Here's the drawing with two shaded views (mm, measured from the low corner). I have some questions. Give positions to 0.01 mm unless a question says otherwise; leave off trailing zeros. Order: outer loops, then holes, each group sorted by start corner. A loop starts at its lowest first (then second) coordinate and runs counter-clockwise, first axis right, second up. Notation, with made-up numbers: (55, -6.5) - (102, -6.5) arc R16 cw to (102, -1.5) - close; hole circle Ø3 at (-35, 19.5). An arc over 180 degrees is marked (long way). Use one line per item in the form item = value. Start each with the question number.
1) For pin 1 (10 mm diameter, centred on y = 25, z = 12.5, fed in from -X); pin 2 (8 mm diameter, centred on y = 42.5, z = 20.5, fed in from +X) (1 decimal); pin 3 (10 mm diameter, centred on x = 45, z = 3, fed in from +Y); pin 4 (8 mm diameter, centred on y = 9.5, z = 17, fed in from -X), each with a flat end and sliding along its axis, tell me the tip position at first contact or that it passes through.
2) Suppose I cut it at A-A, the plane z = 14. Write out the boundary of the cut face in (x, y) (1 decimal), and give its area (3 significant figures).
3) Please list where these lines run through material, in increasing order: probe 1 along X at (y, z) = (29.5, 8.75) (1 decimal); probe 2 along X at (y, z) = (28.5, 14.25); probe 3 along Y at (x, z) = (37.5, 18).
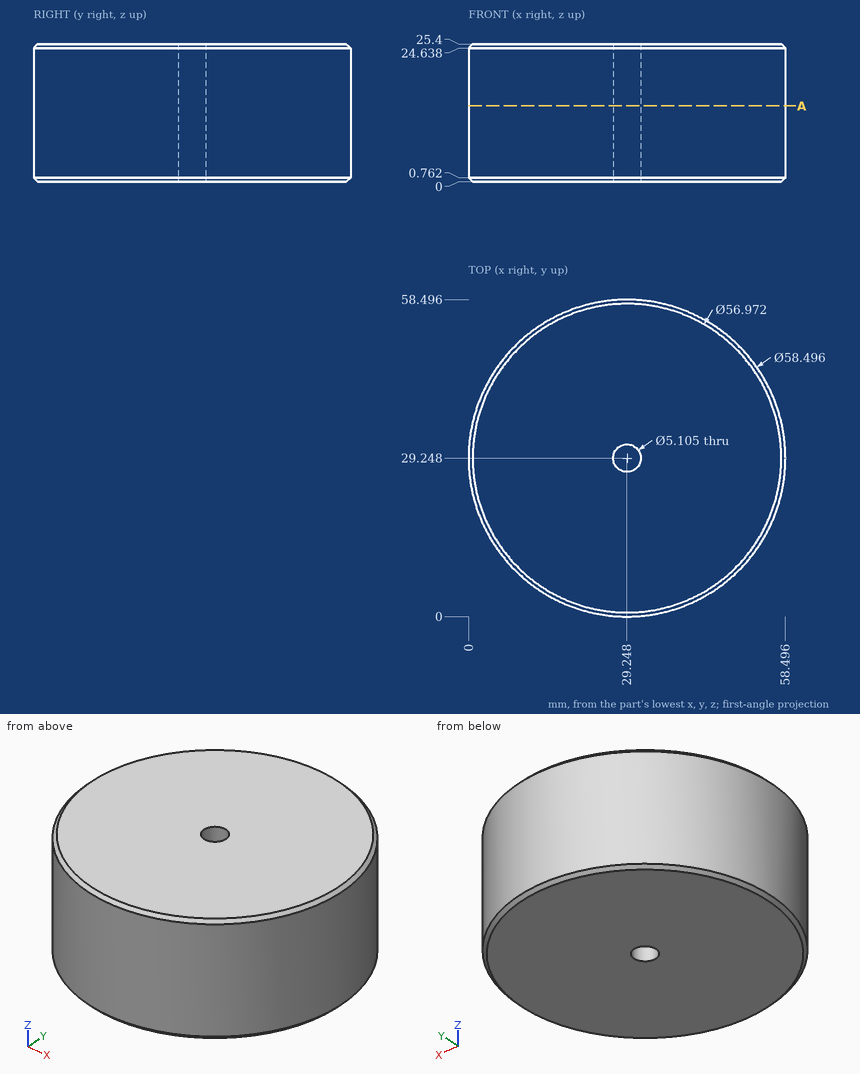
Result sheet:
q1.pin_1 = 0
q1.pin_2 = 57
q1.pin_3 = 56.45
q1.pin_4 = 4.6
q2.outline = circle Ø58.5 at (29.2, 29.2); hole circle Ø5.1 at (29.2, 29.2)
q2.area = 2,670 mm²
q3.probe_1 = 0 to 26.7, 31.8 to 58.5
q3.probe_2 = 0.01 to 26.81, 31.69 to 58.49
q3.probe_3 = 1.19 to 57.31
